Design review of the part built by this model. Coordinates are the model's own, in mm. A direction names the side the tool comes from. Coordinates: 2 decimals unless noted, no trailing zeros. Loops run counter-clockwise (first coordinate to the right, second up) from the corner with the lowest first, then second, coordinate; pieces in that order, holes last. Notation, with made-up numbers: (-3, -18) - (33, -18) arc R15 cw to (33, 1) - close; hole circle Ø6 at (27.5, 50). An arc over 180 degrees is marked (long way). One line per question, with ' | ' between items.
Autodesk Inventor part; units mm, degrees
ref_plane "Work Plane1" through (0, 0, 16.25) normal (0, 0, 1) x (1, 0, 0)
ref_plane "YZ Plane" through (0, 0, 0) normal (1, 0, 0) x (0, 1, 0)
ref_plane "XZ Plane" through (0, 0, 0) normal (0, 1, 0) x (-1, 0, 0)
sketch "Sketch1" plane through (0, 0, 0) normal (0, 1, 0) x (-1, 0, 0)
  circle A0 centre (0, 0) radius 13.75
  circle A1 centre (0, 0) radius 16.25
  dimension "d0" = 27.5
  dimension "d5" = 32.5
sketch "Sketch2" plane through (0, 0, 0) normal (0, 1, 0) x (-1, 0, 0)
  line L0 (21.5, 21.5) -> (-21.5, 21.5)
  line L1 (-21.5, 21.5) -> (-21.5, -21.5)
  line L2 (-21.5, -21.5) -> (21.5, -21.5)
  line L3 (21.5, -21.5) -> (21.5, 21.5)
  point P0 (0, 0)
  dimension "d1" = 43
  dimension "d2" = 43
  dimension "d3" = 21.5
  dimension "d4" = 21.5
extrude "Extrusion1" add sketch "Sketch1" along normal blind 8
sketch "Sketch3" plane through (0, 8, 0) normal (0, 1, 0) x (1, 0, 0)
  line L0 (-17.7413, 16.25) -> (19.579, 16.25) construction
  line L1 (16.25, -18.4481) -> (16.25, 20.2858) construction
  line L2 (-16.25, -20.7099) -> (-16.25, 21.9822) construction
  line L3 (-16.5, 16.25) -> (16.5, 16.25) construction
  line L4 (16.5, 16.25) -> (16.5, 31.25) construction
  line L5 (16.5, 31.25) -> (-16.5, 31.25) construction
  line L6 (-16.5, 31.25) -> (-16.5, 16.25) construction
  circle A0 centre (0, 0) radius 16.25
  line L7 (-16.25, -16.5) -> (-31.25, -16.5) construction
  line L8 (-31.25, -16.5) -> (-31.25, 16.5) construction
  line L9 (-31.25, 16.5) -> (-16.25, 16.5) construction
  line L10 (-16.25, 16.5) -> (-16.25, -16.5) construction
  line L11 (16.25, -16.5) -> (31.25, -16.5) construction
  line L12 (31.25, -16.5) -> (31.25, 16.5) construction
  line L13 (31.25, 16.5) -> (16.25, 16.5) construction
  line L14 (16.25, 16.5) -> (16.25, -16.5) construction
  line L15 (-16.5, -16.5) -> (16.25, -16.5)
  line L16 (16.5, 16.5) -> (16.5, 16.25)
  line L17 (-10, 12.8087) -> (-10, 16.5)
  line L18 (10, 12.8087) -> (10, 16.5)
  line L19 (16.5, 16.5) -> (-10, 16.5)
  line L20 (-16.25, 16.5) -> (-16.5, 16.5)
  line L21 (-16.5, 16.5) -> (-16.5, 16.25)
  line L22 (-16.5, 10) -> (-16.5, -10)
  line L23 (16.4416, -10) -> (16.4416, 10)
  circle A1 centre (0, 0) radius 16.25
  line L24 (-16.5, 10) -> (-12.8087, 10)
  line L25 (12.8087, 10) -> (16.4416, 10)
  line L26 (16.4416, -10) -> (12.8087, -10)
  line L27 (-12.8087, -10) -> (-16.5, -10)
  dimension "d8" = 33
  dimension "d9" = 15
  dimension "d10" = 16.5
  dimension "d11" = 15
  dimension "d12" = 16.5
  dimension "d13" = 33
  dimension "d14" = 16.5
  dimension "d15" = 15
  dimension "d16" = 33
  dimension "d20" = 10
  dimension "d21" = 10
extrude "Extrusion2" add sketch "Sketch3" against normal blind 20 contours A0 L25 L23 L26 | A0 L17 L19 L18 | L27 L22 L24 A0
sketch "Sketch4" plane through (16.4416, 8, 10) normal (1, 0, 0) x (0, 0, -1)
  line L0 (20, -20) -> (0, -20)
  line L1 (-3.75, 0) -> (23.75, 0)
  line L2 (-6.5, -20) -> (26.5, -20)
  line L3 (26.5, -20) -> (26.5, 0)
  line L4 (26.5, 0) -> (-6.5, 0)
  line L5 (-6.5, 0) -> (-6.5, -20)
  line L6 (10, 0) -> (10, -20) construction
  line L7 (2.5, 0) -> (2.5, -20) construction
  line L8 (17.5, 0) -> (17.5, -20) construction
  line L9 (-6.5, -13.5) -> (26.5, -13.5) construction
  line L10 (22.8087, -8) -> (20, -8)
  circle A0 centre (2.5, -13.5) radius 1
  circle A1 centre (17.5, -13.5) radius 1
  point P0 (10, -8)
  dimension "d26" = 33
  dimension "d27" = 20
  dimension "d28" = 16.5
  dimension "d29" = 7.5
  dimension "d30" = 7.5
  dimension "d31" = 5.5
  dimension "d32" = 2
  dimension "d33" = 2
extrude "Extrusion3" cut sketch "Sketch4" against normal through all contours A0 | A1
sketch "Sketch5" plane through (10, 8, -16.5) normal (0, 0, -1) x (-1, 0, 0)
  line L0 (-10.5226, -13.5) -> (32.3111, -13.5) construction
  line L1 (0, -8) -> (-2.8087, -8)
  circle A0 centre (2.5, -13.5) radius 1
  circle A1 centre (17.5, -13.5) radius 1
  point P0 (10, -8)
  dimension "d36" = 5.5
  dimension "d37" = 2
  dimension "d38" = 2
  dimension "d39" = 7.5
  dimension "d40" = 7.5
extrude "Extrusion4" cut sketch "Sketch5" against normal through all
ref_plane "Work Plane1" through (0, 0, 16.25) normal (0, 0, 1) x (1, 0, 0)
sketch "Sketch9" plane through (16.4416, 8, 10) normal (1, 0, 0) x (0, 0, -1)
  line L0 (0, 0) -> (-6.25, 0)
  line L1 (20, -20) -> (0, -20)
  line L2 (0, 0) -> (20, 0)
  line L3 (20, 0) -> (20, -20)
  line L4 (20, -20) -> (0, -20)
  line L5 (0, -20) -> (0, 0)
  circle A0 centre (2.5, -13.5) radius 1
  circle A1 centre (2.5, -13.5) radius 1
  circle A2 centre (17.5, -13.5) radius 1
  circle A3 centre (17.5, -13.5) radius 1
  point P0 (10, -8)
extrude "Extrusion7" add sketch "Sketch9" along normal blind 3
sketch "Sketch10" plane through (10, 8, -16.5) normal (0, 0, -1) x (-1, 0, 0)
  line L0 (-3.75, 0) -> (23.75, 0)
  line L1 (0, -8) -> (0, -20)
  line L2 (19.9113, 0) -> (0, 0)
  line L3 (0, 0) -> (0, -20)
  line L4 (0, -20) -> (19.9113, -20)
  line L5 (19.9113, -20) -> (19.9113, 0)
  circle A0 centre (17.5, -13.5) radius 1
  circle A1 centre (17.5, -13.5) radius 1
  circle A2 centre (2.5, -13.5) radius 1
  circle A3 centre (2.5, -13.5) radius 1
  point P0 (10, -8)
extrude "Extrusion8" add sketch "Sketch10" along normal blind 3
sketch "Sketch11" plane through (-16.5, 8, -10) normal (-1, 0, 0) x (0, 0, 1)
  line L0 (0, 0) -> (-2.8087, 0)
  line L1 (20, -20) -> (0, -20)
  line L2 (0, 0) -> (20, 0)
  line L3 (20, 0) -> (20, -20)
  line L4 (20, -20) -> (0, -20)
  line L5 (0, -20) -> (0, 0)
  circle A0 centre (17.5, -13.5) radius 1
  circle A1 centre (17.5, -13.5) radius 1
  circle A2 centre (2.5, -13.5) radius 1
  circle A3 centre (2.5, -13.5) radius 1
  point P0 (10, -8)
extrude "Extrusion9" add sketch "Sketch11" along normal blind 3
sketch "Sketch6" plane through (0, 0, 16.25) normal (0, 0, 1) x (1, 0, 0)
  line L0 (10, 8) -> (-10, 8)
  line L1 (-10.5, 8) -> (10.5, 8)
  line L2 (10.5, 8) -> (10.5, -23)
  line L3 (10.5, -23) -> (-10.5, -23)
  line L4 (-10.5, -23) -> (-10.5, 8)
  circle A0 centre (-5.7, -21) radius 1
  circle A1 centre (5.7, -21) radius 1
  point P0 (0, 0)
  dimension "d44" = 21
  dimension "d45" = 10.5
  dimension "d46" = 31
  dimension "d47" = 2
  dimension "d48" = 2
  dimension "d49" = 4.8
  dimension "d50" = 4.8
  dimension "d51" = 2
  dimension "d52" = 2
sketch "Sketch7" plane through (16.4416, 8, 10) normal (1, 0, 0) x (0, 0, -1)
  line L0 (0, -8) -> (0, -20)
  line L1 (20, -8) -> (20, 0)
  line L2 (0, -20) -> (20, -20)
  line L3 (20, -20) -> (20, 0)
  line L4 (20, 0) -> (0, 0)
  line L5 (0, 0) -> (0, -20)
  circle A0 centre (2.5, -13.5) radius 1
  circle A1 centre (2.5, -13.5) radius 1
  circle A2 centre (17.5, -13.5) radius 1
  circle A3 centre (17.5, -13.5) radius 1
  point P0 (10, -8)
properties part number "Battery and PI holder"
Q1. Draft analysis for pull direction Z (two halves, no side actions). For faces 1 (the cylindrical face through (17.228, -5.8, -8.454)), 2 (the flat face through (-16, -2, 10)), 3 (the cylindrical face through (11.47, 3.94, -11.51)), state which applies: +Z half, -Z half, draft (parallel to the pull), parting line (faces both ways), or undercut.
Returned:
face 1: undercut | face 2: +Z half | face 3: -Z half
Q2. For pin 1 (3.5 mm diameter, centred on x = -14.5, y = 1, fed in from +Z); pin 2 (1.8 mm diameter, centred on y = -3.5, z = -14, fed in from -X); pin 3 (7.5 mm diameter, centred on x = -15.5, y = -5.5, fed in from -Z), all flat-tipped, find the tip position at first contact; note any pin that passes through.
Returned:
pin 1: stops at z = 10.07 | pin 2: stops at x = -10 | pin 3: stops at z = -10
Q3. Take a section at C-C (x = 7.5). Give the boundary of the cut face in (y, z), plus the area to 3 significant figures.
Returned:
outline: (-12, -19.5) - (-6.5, -19.5) - (-6.5, -14.42) - (-12, -14.42) - close; (-4.5, -19.5) - (8, -19.5) - (8, -11.52) - (0, -11.52) - (0, -14.42) - (-4.5, -14.42) - close; (0, 11.52) - (8, 11.52) - (8, 14.42) - (0, 14.42) - close | area: 138 mm²
Q4. To check wall thickness, follow line 1 along Y through (x, z) = (15.3, 7.5); line 2 along X through (y, z) = (3.5, -5.5); line 3 along X through (y, z) = (-0.5, -13.5). State the ranges of each line that lie inside material, in increasing order.
Returned:
line 1: y = -12 to -6.5, -4.5 to 8 | line 2: x = -19.5 to -12.6, 12.6 to 19.44 | line 3: x = -10 to -9.05, 9.05 to 10
Q5. Take a section at B-B (y = 3.25). Give the boundary of the cut face in (x, z).
Returned:
outline: (-19.5, -10) - (-12.81, -10) arc R16.25 ccw to (-10, -12.81) - (-10, -16.5) - (-9.91, -16.5) - (-9.91, -19.5) - (10, -19.5) - (10, -12.81) arc R16.25 ccw to (12.81, -10) - (19.44, -10) - (19.44, 10) - (12.81, 10) arc R16.25 ccw to (-12.81, 10) - (-19.5, 10) - close; hole circle Ø27.5 at (0, 0)
Q6. Take a section at D-D (z = -7.5). Give the boundary of the cut face in (x, y), plus the area to 3 significant figures.
Returned:
outline: (-19.5, -12) - (-14.42, -12) - (-14.42, -6.5) - (-19.5, -6.5) - close; (-19.5, -4.5) - (-14.42, -4.5) - (-14.42, 0) - (-11.52, 0) - (-11.52, 8) - (-19.5, 8) - close; (11.52, 0) - (14.42, 0) - (14.42, -4.5) - (19.44, -4.5) - (19.44, 8) - (11.52, 8) - close; (14.42, -12) - (19.44, -12) - (19.44, -6.5) - (14.42, -6.5) - close | area: 228 mm²
Q7. Take a section at A-A (z = 0). Give the boundary of the cut face in (x, y), plus the area to 3 significant figures.
Returned:
outline: (-19.5, -12) - (-16.25, -12) - (-16.25, 0) - (-13.75, 0) - (-13.75, 8) - (-19.5, 8) - close; (13.75, 0) - (16.25, 0) - (16.25, -12) - (19.44, -12) - (19.44, 8) - (13.75, 8) - close | area: 169 mm²
Q8. Tool access review of faces 4 (the flat face through (12.1, 0, 7.3)), 5 (the flat face through (-16, -2, -10)), 6 (the flat face through (16, -2, 10)), 7 (the cylindrical face through (0.15, -5.92, -16.25)), 8 (the flat face through (16, -2, -10)): name each direction out of +Z, -Z, +X, -X, +Y, -Y from which nothing blocks a thin tool from reaching the whole face with its end or side.
Returned:
face 4: -Y | face 5: -Z, -X, +Y, -Y | face 6: +Z, +X, +Y, -Y | face 7: +Z, -Y | face 8: -Z, +X, +Y, -Y
